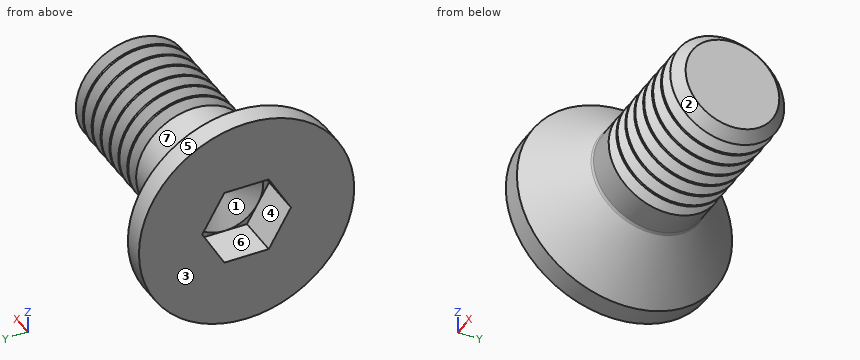
```python
from build123d import *

# Parameters (mm, degrees)
FILLET1_R       = 0.1
HEX_2_DEPTH     = 1.1
THDSCHPAT_COUNT = 7
THDSCHPAT_PITCH = 0.448571429


with BuildPart() as part:
    # BodySke → BaseBody (revolve)
    with BuildSketch(Plane.XY, mode=Mode.PRIVATE) as basebody_sk:
        Polygon((0, 0), (0, 2.8), (0.56, 2.8), (1.86, 1.5), (5.7195, 1.5), (6, 1.2195), (6, 0), align=None)
    revolve(basebody_sk.sketch.rotate(Axis((0, 0, 0), (1, 0, 0)), 90), axis=Axis((0, 0, 0), (1, 0, 0)))

    # Fillet1
    fillet1_edges = [part.edges().sort_by_distance(p)[0] for p in [
        (1.86, 0, -1.5),
    ]]
    fillet(fillet1_edges, radius=FILLET1_R)

    # Sketch2 → PreBroach (revolve, cut)
    with BuildSketch(Plane.XY, mode=Mode.PRIVATE) as prebroach_sk:
        Polygon((0, 1), (1.1, 1), (1.677350269, 0), (0, 0), align=None)
    revolve(prebroach_sk.sketch.rotate(Axis((0, 0, 0), (1, 0, 0)), 90), axis=Axis((0, 0, 0), (1, 0, 0)), mode=Mode.SUBTRACT)

    # Sketch3 → Hex 2 (cut)
    with BuildSketch(Plane.ZY):
        Polygon((-1, -0.577350269), (-1, 0.577350269), (0, 1.154700538), (1, 0.577350269), (1, -0.577350269), (0, -1.154700538), align=None)
    extrude(amount=-HEX_2_DEPTH, mode=Mode.SUBTRACT)

    # ThdSchSke → ThreadSchematic (revolve, cut)
    with BuildSketch(Plane.XY, mode=Mode.PRIVATE) as threadschematic_sk:
        Polygon((2.860001, -1.2195), (2.663592786, -1.5), (2.663592786, -1.875), (3.056409214, -1.875), (3.056409214, -1.5), align=None)
    threadschematic = revolve(threadschematic_sk.sketch.rotate(Axis((-3.175, 0, 0), (1, 0, 0)), 270), axis=Axis((-3.175, 0, 0), (1, 0, 0)), mode=Mode.SUBTRACT)

    # ThdSchPat: ThreadSchematic ×7
    with Locations(*[(i * THDSCHPAT_PITCH, 0, 0) for i in range(1, THDSCHPAT_COUNT)]):
        add(threadschematic, mode=Mode.SUBTRACT)


solid = part.part
```
The model under review builds one solid part; all positions refer to its coordinate system, in mm. Face numbers are marked on the shaded views. A direction names the side the tool comes from. Round coordinates to 2 decimals unless told otherwise and drop trailing zeros. Answer in a Markdown table with one row per item.
(1) Machinability: for the marked faces 5, 6 and 7, which of the approach directions +Z, -Z, +X, -X, +Y, -Y give a long, thin tool a straight path to every point of the face, cutting with its end or side? Answer none if there is none.
Result set:
| item | result |
|---|---|
| face 5 | +X, -X |
| face 6 | -X |
| face 7 | +X |
(2) Clearance check with a flat-ended pin moving along its axis: P1, Ø1.5, axis at x = 4, z = -1.5, coming from the -Y side. State where the tip first meets the part, or that it passes through.
Result set:
| item | result |
|---|---|
| P1 | stops at y = -1.3 |
(3) Take a section at A-A on z = 1.4. Count the separate pieces of the cut face and the enclosed holes in it, plus the area to 3 significant figures.
Result set:
| item | result |
|---|---|
| separate pieces | 8 |
| enclosed holes | 0 |
| area | 8.82 mm2 |
(4) Mouldability with a two-part tool opening along Z and no side actions: class the marked faces 1, 2, 3 and 4 as released by +Z, released by -Z, zero draft, split by the parting line, or undercut.
Result set:
| item | result |
|---|---|
| face 1 | undercut |
| face 2 | split by the parting line |
| face 3 | zero draft |
| face 4 | undercut |
(5) For line 1 (X direction, y = -0.45, z = 0.05); line 2 (Z direction, x = 5.2, y = 0.15); line 3 (X direction, y = -1.8, z = -1.8), list the stretches that pass through material, from the lowest coordinate up. Write a range as from..to.
Result set:
| item | result |
|---|---|
| line 1 | x = 1.42..6 |
| line 2 | z = -1.35..1.35 |
| line 3 | x = 0..0.81 |
